Geometry check sheet. Reference: the model listing, model coordinates, mm. Face numbers are marked on the shaded views. A direction names the side the tool comes from. Round coordinates to 2 decimals unless told otherwise and drop trailing zeros. Write each loop counter-clockwise with the first axis right and the second up, starting at its lowest first coordinate (ties: lowest second). Pieces come first, ordered by that corner, then holes.
Item 1: Cross-section at B-B (y = 76). Enter the section's corners in (x, z).
Item 2: Access from +Z, -Z, +X, -X, +Y, -Y to the whole of each face (thin tool, end or side, straight path). Record for the marked faces 1 and 2.
Item 3: Scan lines: probe 1 along Y at (x, z) = (3.75, -1.75); probe 2 along Y at (x, z) = (-0.5, 2.5); probe 3 along X at (y, z) = (64, -0.5). Record each from-to range of solid material in increasing order.
Item 4: Depth check by flat-ended pin: P1, Ø3, axis at y = 78, z = 0, coming from the +X side; P2, Ø1.5, axis at x = -2.5, y = 14, coming from the +Z side; P3, Ø2.5, axis at x = 1, z = 0, coming from the -Y side. Enter the tip coordinate at first touch or a pass-through.
Item 5: Cross-section at A-A (z = 0). Enter the section's corners in (x, y).
Autodesk Inventor part; units mm, degrees
ref_plane "YZ Plane" through (0, 0, 0) normal (1, 0, 0) x (0, 1, 0)
ref_plane "XZ Plane" through (0, 0, 0) normal (0, 1, 0) x (-1, 0, 0)
ref_plane "XY Plane" through (0, 0, 0) normal (0, 0, 1) x (1, 0, 0)
sketch "Sketch1" plane through (0, 0, 0) normal (0, 1, 0) x (-1, 0, 0)
  circle A0 centre (0, 0) radius 5
  circle A1 centre (0, 0) radius 3
  dimension "d0" = 10
  dimension "d1" = 6
extrude "Extrusion1" add sketch "Sketch1" along normal blind 100 contours A1
extrude "Extrusion2" add sketch "Sketch1" along normal blind 6
fillet "Fillet1" radius 0.3 1 edges at (5, 0, 0)
fillet "Fillet2" radius 0.3 1 edges at (5, 6, 0)
sketch "Sketch2" plane through (0, 0, 0) normal (0, -1, 0) x (1, 0, 0)
  line L0 (0, -2.8868) -> (-2.5, -1.4434)
  line L1 (-2.5, -1.4434) -> (-2.5, 1.4434)
  line L2 (-2.5, 1.4434) -> (0, 2.8868)
  line L3 (0, 2.8868) -> (2.5, 1.4434)
  line L4 (2.5, 1.4434) -> (2.5, -1.4434)
  line L5 (2.5, -1.4434) -> (0, -2.8868)
  point P0 (0, 0)
  point P1 (0, 0)
  dimension "d8" = 5
extrude "Extrusion3" cut sketch "Sketch2" against normal blind 1.3
thread "Thread1"
properties part number "m6_bolt100mm"
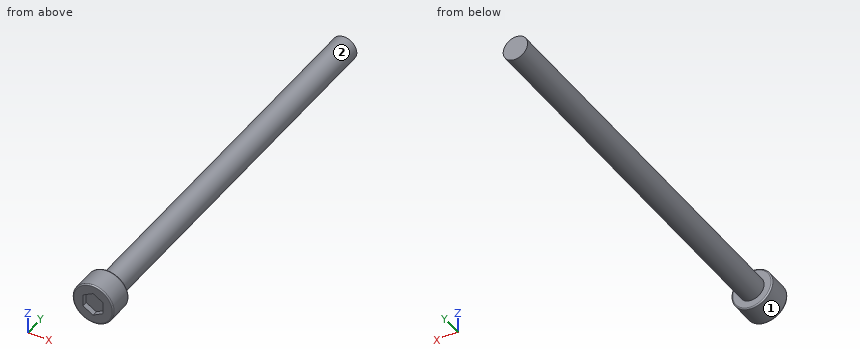
Resolved:
1. outline: circle Ø6 at (0, 0)
2. face 1: +Y, -Y
2. face 2: +Y
3. probe 1: y = 0 to 6
3. probe 2: y = 1.3 to 100
3. probe 3: x = -2.96 to 2.96
4. P1: stops at x = 3
4. P2: stops at z = 2.44
4. P3: stops at y = 1.3
5. outline: (-5, 0.3) arc R0.3 ccw to (-4.7, 0) - (-2.5, 0) - (-2.5, 1.3) - (2.5, 1.3) - (2.5, 0) - (4.7, 0) arc R0.3 ccw to (5, 0.3) - (5, 5.7) arc R0.3 ccw to (4.7, 6) - (3, 6) - (3, 100) - (-3, 100) - (-3, 6) - (-4.7, 6) arc R0.3 ccw to (-5, 5.7) - close
